Design review of the part built by this model. Coordinates are the model's own, in mm. Face numbers are marked on the shaded views. Coordinates: 2 decimals unless noted, no trailing zeros. Write each loop counter-clockwise with the first axis right and the second up, starting at its lowest first coordinate (ties: lowest second). Pieces come first, ordered by that corner, then holes. Notation, with made-up numbers: (32, 77.5) -> (78, 77.5) arc R15 ccw to (78, 101.5) -> close; hole circle Ø9 at (66, 28.5). An arc over 180 degrees is marked (long way). Answer in a Markdown table with one row per item. Add a question column.
Item 1: Take a section at A-A, the plane y = 3.5. Write out the cut boundary in (x, z).
Item 2: To check wall thickness, follow line 1 (X direction, y = 3.5, z = 1.95); line 2 (X direction, y = 3.25, z = 0.4); line 3 (X direction, y = -0.25, z = 0.35). State the ranges of each line that lie inside material, in increasing order.
Item 3: Take a section at D-D, the plane y = -0.5. Write out the cut boundary in (x, z).
Item 4: Draft analysis for pull direction X (two halves, no side actions). For the marked faces 1, 2 and 3, state which applies: released by +X, released by -X, zero draft, split by the parting line, or undercut.
Item 5: Take a section at B-B, the plane z = 0.35. Write out the cut boundary in (x, y).
Item 6: Take a section at C-C, the plane x = 9.25. Write out the cut boundary in (y, z), and give its area (3 significant figures).
from build123d import *

# Parameters (mm, degrees)
BOSS_EXTRUDE1_DEPTH = 3


with BuildPart() as part:
    # Sketch1 → Boss-Extrude1 (new body)
    with BuildSketch(Plane(origin=(0, 0, 0), x_dir=(0, 1, 0), z_dir=(0, 0, 1))):
        with BuildLine():
            Line((-2.122941602, 14.254932242), (-2.122941602, -10.553285524))
            ThreePointArc((-2.122941602, -10.553285524), (-1.244261946, -12.674605867), (0.877058398, -13.553285524))
            Line((0.877058398, -13.553285524), (3.877058398, -13.553285524))
            Line((3.877058398, -13.553285524), (3.006420494, -11.983925105))
            ThreePointArc((3.006420494, -11.983925105), (2.340422166, -8.716396804), (3.877058398, -5.756828581))
            Line((3.877058398, -5.756828581), (3.877058398, 10.86753602))
            Line((3.877058398, 10.86753602), (-2.122941602, 14.254932242))
        make_face()
    extrude(amount=BOSS_EXTRUDE1_DEPTH)


solid = part.part
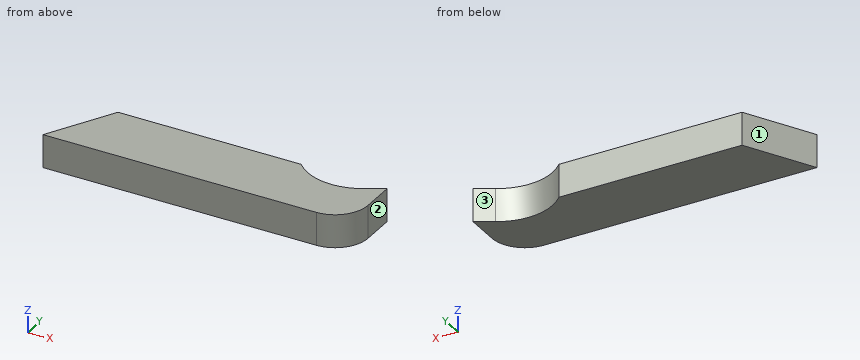
Answers:
| question | item | result |
|---|---|---|
| 1 | outline | (-11.08, 0) -> (6.15, 0) -> (6.15, 3) -> (-11.08, 3) -> close; (12.87, 0) -> (13.55, 0) -> (13.55, 3) -> (12.87, 3) -> close |
| 2 | line 1 | x = -11.08 to 6.15, 12.87 to 13.55 |
| 2 | line 2 | x = -11.22 to 6.47, 12.42 to 13.55 |
| 2 | line 3 | x = -13.2 to 13.33 |
| 3 | outline | (-13.34, 0) -> (13.22, 0) -> (13.22, 3) -> (-13.34, 3) -> close |
| 4 | face 1 | released by -X |
| 4 | face 2 | released by +X |
| 4 | face 3 | undercut |
| 5 | outline | (-14.25, -2.12) -> (10.55, -2.12) arc R3 ccw to (13.55, 0.88) -> (13.55, 3.88) -> (11.98, 3.01) arc R5 cw to (5.76, 3.88) -> (-10.87, 3.88) -> close |
| 6 | outline | (-2.12, 0) -> (2.29, 0) -> (2.29, 3) -> (-2.12, 3) -> close |
| 6 | area | 13.3 mm^2 |
